Source: three-view drawing plus pictorial views. Frame: mm from the lowest corner of the part. A direction names the side the tool comes from. Coordinates: 2 decimals unless noted, no trailing zeros. Loops run counter-clockwise (first coordinate to the right, second up) from the corner with the lowest first, then second, coordinate; pieces in that order, holes last. Notation, with made-up numbers: (11, -29.75) - (18, -29.75) arc R27 cw to (18, -4.75) - close; hole circle Ø6 at (1, -17.5). An arc over 180 degrees is marked (long way). Return JSON: item names as keys, results as strings.
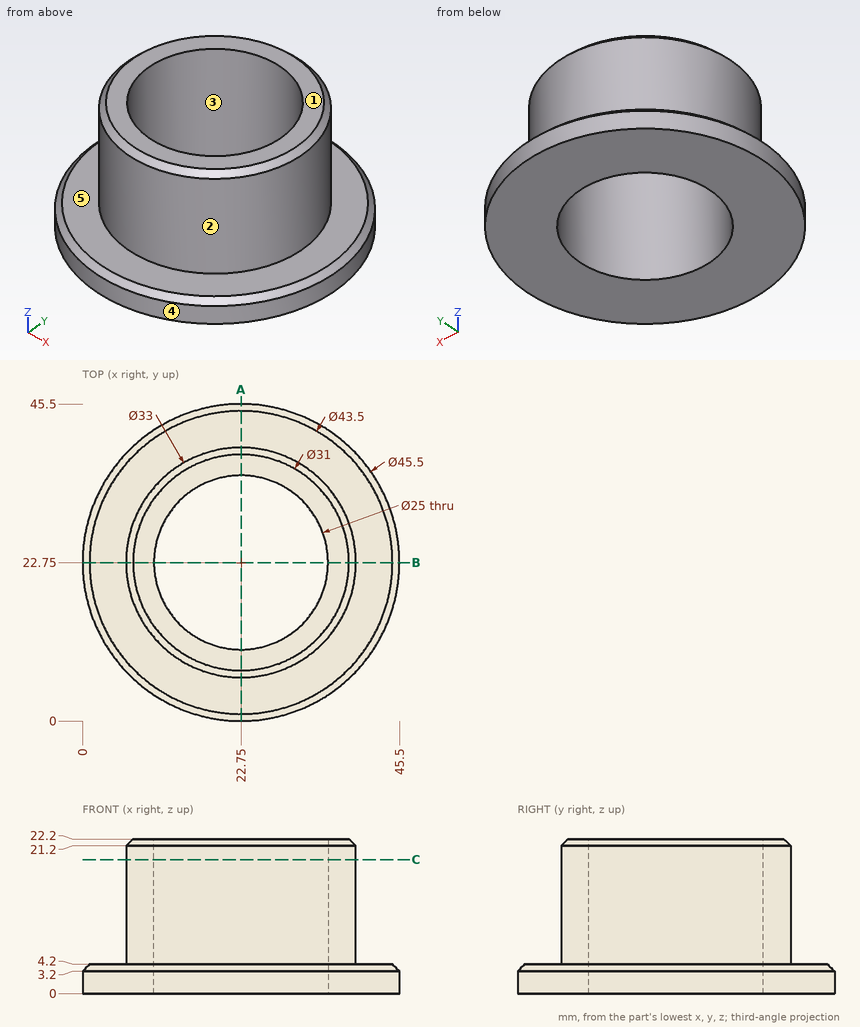
Item 1: Ray query, probe 1 along Y at (x, z) = (22.75, 5); probe 2 along Z at (x, y) = (3, 29.5); probe 3 along X at (y, z) = (19.5, 19.25). Return the intervals inside material, ascending. Write a range as from..to.
Worked out:
{"probe 1": "6.25..10.25, 35.25..39.25", "probe 2": "0..4.2", "probe 3": "6.57..10.68, 34.82..38.93"}
Item 2: Mould query, pull axis Y, two halves, no side actions, for the marked faces 1, 2 and 3. Classes: +Y half, -Y half, draft (parallel to the pull), parting line (faces both ways), or undercut.
Worked out:
{"face 1": "draft", "face 2": "parting line", "face 3": "undercut"}
Item 3: Section query A-A, the plane x = 22.75. Return loops of the section in (y, z).
Worked out:
{"outline": "(0, 0) - (10.25, 0) - (10.25, 22.2) - (7.25, 22.2) - (6.25, 21.2) - (6.25, 4.2) - (1, 4.2) - (0, 3.2) - close; (35.25, 0) - (45.5, 0) - (45.5, 3.2) - (44.5, 4.2) - (39.25, 4.2) - (39.25, 21.2) - (38.25, 22.2) - (35.25, 22.2) - close"}
Item 4: Section query C-C, the plane z = 19.25. Return loops of the section in (x, y).
Worked out:
{"outline": "circle Ø33 at (22.75, 22.75); hole circle Ø25 at (22.75, 22.75)"}
Item 5: First-contact query: pin 1 Ø6 at (x, y) = (6.5, 8.5) entering from +Z; pin 2 Ø12 at (y, z) = (37.5, 20) entering from +X; pin 3 Ø6 at (x, z) = (9, 2.5) entering from +Y; pin 4 Ø22.5 at (x, y) = (22.75, 22.75) entering from +Z. Flat tips, straight axial feed; report the tip coordinate or a pass-through.
Worked out:
{"pin 1": "z = 4.2", "pin 2": "x = 36.74", "pin 3": "y = 42.8", "pin 4": "through"}
Item 6: Reachability of the marked faces 4 and 5 from +Z, -Z, +X, -X, +Y, -Y: full face, straight path, thin tool, end or side. Return the list, or none.
Worked out:
{"face 4": "+Z, -Z", "face 5": "+Z"}
